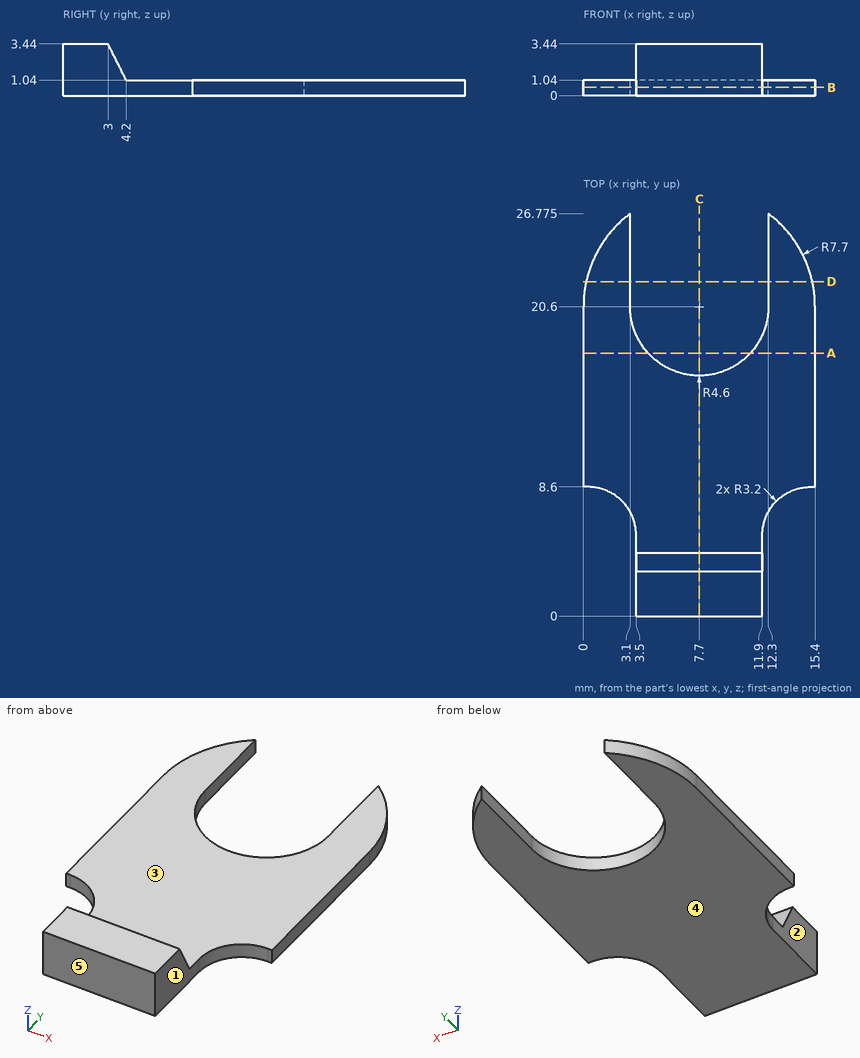
Design review of the part shown in the three views and the two pictorial views. Dimensions are in mm from the part's minimum x, y and z. A direction names the side the tool comes from. Give positions to 0.01 mm unless a question says otherwise; leave off trailing zeros. Loops run counter-clockwise (first coordinate to the right, second up) from the corner with the lowest first, then second, coordinate; pieces in that order, holes last. Notation, with made-up numbers: (86, 88.25) -> (130, 88.25) arc R15 ccw to (130, 106.25) -> close; hole circle Ø7 at (40.5, 14). An arc over 180 degrees is marked (long way). Put each result on its own line as item: value. Start each with the question number.
1. We need section D-D on y = 22.25. State the section outline as (x, z) points.
2. We need section C-C on x = 7.7. State the section outline as (y, z) points, then the cut area to 3 significant figures.
3. Wall thickness on probe 1 along Z at (x, y) = (10.5, 8.5); probe 2 along X at (y, z) = (19, 0.3); probe 3 along X at (y, z) = (25, 0.7): over which ranges is each line inside the solid? List them lowest first.
4. We need section A-A on y = 17.5. State the section outline as (x, z) points.
5. We need section B-B on z = 0.55. State the section outline as (x, y) points (3 decimals).
6. Clearance check with flat-ended pins moving along their axes: P1, Ø2, axis at x = 1.5, y = 23.5, coming from the -Z side; P2, Ø2, axis at x = 13, z = 3, coming from the +Y side; P3, Ø1.1, axis at y = 25, z = 1, coming from the -X side; P4, Ø0.8, axis at y = 25, z = 0.5, coming from the +X side. State where each tip first meets the part, or that it passes through.
7. For the marked faces 1, 2, 3, 4 and 5, list the 3-axis set-ups (+Z, -Z, +X, -X, +Y, -Y) from which the entire face can be reached by the end or side of a thin tool; tool diameter is ignored.
Determined:
1. outline: (0.18, 0) -> (3.1, 0) -> (3.1, 1.04) -> (0.18, 1.04) -> close; (12.3, 0) -> (15.22, 0) -> (15.22, 1.04) -> (12.3, 1.04) -> close
2. outline: (0, 0) -> (16, 0) -> (16, 1.04) -> (4.2, 1.04) -> (3, 3.44) -> (0, 3.44) -> close
2. area: 25.3 mm^2
3. probe 1: 0 to 1.04
3. probe 2: 0 to 3.39, 12.01 to 15.4
3. probe 3: 1.38 to 3.1, 12.3 to 14.02
4. outline: (0, 0) -> (4.3, 0) -> (4.3, 1.04) -> (0, 1.04) -> close; (11.1, 0) -> (15.4, 0) -> (15.4, 1.04) -> (11.1, 1.04) -> close
5. outline: (0, 8.6) -> (0.3, 8.6) arc R3.2 cw to (3.5, 5.4) -> (3.5, 0) -> (11.9, 0) -> (11.9, 5.4) arc R3.2 cw to (15.1, 8.6) -> (15.4, 8.6) -> (15.4, 20.6) arc R7.7 ccw to (12.3, 26.775) -> (12.3, 20.6) arc R4.6 cw to (3.1, 20.6) -> (3.1, 26.775) arc R7.7 ccw to (0, 20.6) -> close
6. P1: z = 0
6. P2: through
6. P3: x = 1.03
6. P4: x = 14.28
7. face 1: +Z, -Z, +X, -Y
7. face 2: +Z, -Z, -X, -Y
7. face 3: +Z, +X, -X, +Y
7. face 4: -Z, +X, -X, +Y, -Y
7. face 5: +Z, -Z, +X, -X, -Y
